from build123d import *

# Parameters (mm, degrees)
F0_R     = 9.525
F1_DEPTH = 15.875
F2_R     = 3.96875
F3_DEPTH = 15.876
F4_R     = 6.223
F4_R_2   = 3.96875
F5_DEPTH = 8.382
F6_SIZE  = 0.254
F7_R     = 3.96875
F8_DEPTH = 10.5250001002


with BuildPart() as f1:
    # F0 (on Front) → F1 (new body)
    with BuildSketch(Plane.XZ):
        Circle(F0_R)
    extrude(amount=F1_DEPTH)

    # F2 (on face) → F3 (cut, through all)
    with BuildSketch(Plane.XZ.offset(15.875)):
        Circle(F2_R)
    extrude(amount=-F3_DEPTH, mode=Mode.SUBTRACT)

    # F4 (on face) → F5 (cut)
    with BuildSketch(Plane.XZ.offset(15.875)):
        Circle(F4_R)
        Circle(F4_R_2, mode=Mode.SUBTRACT)
    extrude(amount=-F5_DEPTH, mode=Mode.SUBTRACT)

    # F6
    f6_edges = [f1.edges().sort_by_distance(p)[0] for p in [
        (-9.525, -15.875, 0),
        (-9.525, 0, 0),
    ]]
    chamfer(f6_edges, length=F6_SIZE)

    # F7 (on Top) → F8 (cut, up to face)
    with BuildSketch(Plane.XY):
        with Locations((0, -10.414)):
            Circle(F7_R)
    extrude(amount=F8_DEPTH, mode=Mode.SUBTRACT)


solid = f1.part
Can you work these out from the model? Positions are in its coordinate system, mm. A direction names the side the tool comes from. Coordinates: 2 decimals unless noted, no trailing zeros. Write each loop counter-clockwise with the first axis right and the second up, starting at its lowest first coordinate (ties: lowest second). Pieces come first, ordered by that corner, then holes. Notation, with made-up numbers: (-11, 8) - (31, 8) arc R23 cw to (31, 19) - close; hole circle Ø7 at (53.5, -12.5). An arc over 180 degrees is marked (long way). Return JSON: item names as keys, results as strings. Group by question number.
Item 1: If we section it at A-A (z = 0): Write out the boundary of the cut face in (x, y) (3 decimals), then the cut area to 3 significant figures.
Item 2: We'd pull the mould along Y, two halves only. Please class faces 1 (the face through (-0.86, -3.799, -3.874)), 2 (the face through (-0.1, -7.493, -4.2)), 3 (the face through (2.134, -7.068, 6.914)): pulls with the +Y half, pulls with the -Y half, needs draft (parallel to the pull), parting line crosses it, or undercut.
Item 3: If we section it at B-B (x = 0): Write out the boundary of the cut face in (y, z) (3 decimals).
Item 4: Which directions (+Z, -Z, +X, -X, +Y, -Y) give clear straight access to the entire face, cutting with the end or side of a thin tool? Please do faces 4 (the face through (-1.349, -11.743, -6.075)), 5 (the face through (4, 0, -2)).
Item 5: If we section it at D-D (y = -12): Write out the boundary of the cut face in (x, z) (3 decimals), then the cut area to 3 significant figures.
Item 6: Please list where these lines run through material, in increasing order: probe 1 along Z at (x, y) = (0, -2.5) (3 decimals); probe 2 along Y at (x, z) = (-4.75, -3.5); probe 3 along X at (y, z) = (-8.25, 0.75).
Item 7: I'm going to push flat-ended pins straight in: pin 1 Ø4 at (y, z) = (-2, 2.5) entering from -X; pin 2 Ø4 at (x, y) = (-7.5, -6) entering from +Z; pin 3 Ø1 at (x, y) = (-3.5, -3.5) entering from -Z. Where does each tip first touch, or does it pass through?
Return value:
{
 "1": {"outline": "(-9.525, -15.621) - (-9.271, -15.875) - (-6.223, -15.875) - (-6.223, -7.493) - (-3.969, -7.493) - (-3.969, 0) - (-9.271, 0) - (-9.525, -0.254) - close; (3.969, -7.493) - (6.223, -7.493) - (6.223, -15.875) - (9.271, -15.875) - (9.525, -15.621) - (9.525, -0.254) - (9.271, 0) - (3.969, 0) - close", "area": "138 mm^2"},
 "2": {"face 1": "needs draft", "face 2": "pulls with the -Y half", "face 3": "undercut"},
 "3": {"outline": "(-15.875, -9.271) - (-15.621, -9.525) - (-0.254, -9.525) - (0, -9.271) - (0, -3.969) - (-7.493, -3.969) - (-7.493, -6.223) - (-15.875, -6.223) - close; (-15.875, 6.223) - (-14.383, 6.223) - (-14.383, 9.525) - (-15.621, 9.525) - (-15.875, 9.271) - close; (-6.445, 3.969) - (0, 3.969) - (0, 9.271) - (-0.254, 9.525) - (-6.445, 9.525) - close"},
 "4": {"face 4": "-Y", "face 5": "+Z, -Z, +X, -X, +Y"},
 "5": {"outline": "(-3.638, 5.049) - (-3.638, 8.803) arc R9.525 ccw (long way) to (3.638, 8.803) - (3.638, 5.049) arc R6.223 cw (long way) to start", "area": "138 mm^2"},
 "6": {"probe 1": "z = -9.525 to -3.969, 3.969 to 9.525", "probe 2": "y = -7.49 to 0", "probe 3": "x = -9.5 to -6.18, 6.18 to 9.5"},
 "7": {"pin 1": "stops at x = -9.51", "pin 2": "stops at z = 7.78", "pin 3": "stops at z = -9.04"}
}
